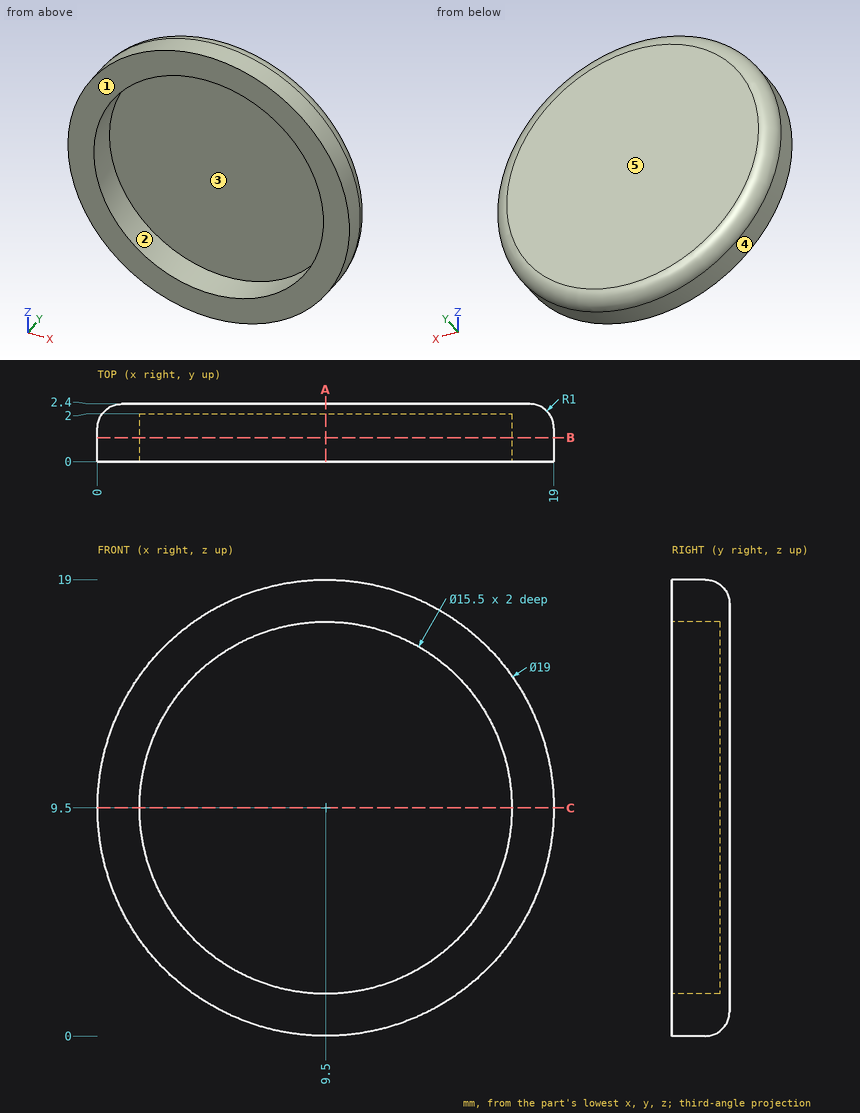
Geometry check sheet. Reference: drawing and pictorial views, mm from the part's lowest x, y, z. A direction names the side the tool comes from. Round coordinates to 2 decimals unless told otherwise and drop trailing zeros. Loops run counter-clockwise (first coordinate to the right, second up) from the corner with the lowest first, then second, coordinate; pieces in that order, holes last. Notation, with made-up numbers: (-28.75, 88.5) - (-0.75, 88.5) arc R29 ccw to (-0.75, 109.5) - close; hole circle Ø11 at (87.25, 80). An arc over 180 degrees is marked (long way). Answer as CSV lines item,"result".
(1) Cross-section at B-B, the plane y = 1. Enter the section's corners in (x, z), and give its area (3 significant figures).
Output values:
outline,"circle Ø19 at (9.5, 9.5); hole circle Ø15.5 at (9.5, 9.5)"
area,"94.8 mm²"
(2) Set-up check for the marked faces 1 and 2: record each of +Z, -Z, +X, -X, +Y, -Y from which the full face is reachable in a straight line by a thin tool's end or side.
Output values:
face 1,"+Z, -Z, +X, -X, -Y"
face 2,"-Y"
(3) Depth check by flat-ended pin: pin 1 Ø8 at (x, z) = (11, 9) entering from -Y. Enter the tip coordinate at first touch or a pass-through.
Output values:
pin 1,"stops at y = 2"
(4) Release check for a two-part mould opening along X. For the marked faces 3, 4 and 5 record: released by +X, released by -X, zero draft, split by the parting line, or undercut.
Output values:
face 3,"undercut"
face 4,"split by the parting line"
face 5,"zero draft"
(5) Cross-section at A-A, the plane x = 9.5. Enter the section's corners in (y, z), and give its area (3 significant figures).
Output values:
outline,"(0, 0) - (1.4, 0) arc R1 ccw to (2.4, 1) - (2.4, 18) arc R1 ccw to (1.4, 19) - (0, 19) - (0, 17.25) - (2, 17.25) - (2, 1.75) - (0, 1.75) - close"
area,"14.2 mm²"
(6) Material ranges on line 1 along Z through (x, y) = (9.5, 0.55); line 2 along Y through (x, z) = (15.25, 13.5); line 3 along Z through (x, y) = (5.5, 1.9), recorded low to high.
Output values:
line 1,"z = 0 to 1.75, 17.25 to 19"
line 2,"y = 2 to 2.4"
line 3,"z = 1.03 to 2.86, 16.14 to 17.97"
(7) Cross-section at C-C, the plane z = 9.5. Enter the section's corners in (x, y).
Output values:
outline,"(0, 0) - (1.75, 0) - (1.75, 2) - (17.25, 2) - (17.25, 0) - (19, 0) - (19, 1.4) arc R1 ccw to (18, 2.4) - (1, 2.4) arc R1 ccw to (0, 1.4) - close"
